Geometry: final body of the model. Coordinates: model frame, mm. Face numbers are marked on the shaded views. A direction names the side the tool comes from. Give positions to 0.01 mm unless a question says otherwise; leave off trailing zeros. Write each loop counter-clockwise with the first axis right and the second up, starting at its lowest first coordinate (ties: lowest second). Pieces come first, ordered by that corner, then holes.
Q1. Line query: line 1 (X direction, y = 0, z = 16.25); line 2 (Y direction, x = -2, z = 49); line 3 (Y direction, x = 0, z = 36). Output: solid intervals per line, ascending.
Q2. Section B-B (y = -64). Return the cut outline in (x, z).
Q3. Pin query (flat end, axial travel): pin 1 Ø22 at (x, z) = (-65, 62.5) entering from -Y; pin 2 Ø3 at (x, z) = (-22.5, 46.5) entering from +Y; pin 3 Ø13 at (x, y) = (50, 50) entering from +Z; pin 4 Ø1 at (x, y) = (-41.5, -2) entering from -Z. Return the tip coordinate at first contact, or that it passes through.
Q4. Mould query, pull axis X, two halves, no side actions, for the marked faces 1, 2, 3 and 4. Classes: +X half, -X half, draft (parallel to the pull), parting line (faces both ways), or undercut.
Q5. Section A-A (x = -91.5). Return the cut outline in (y, z), plus the area to 3 significant figures.
Q6. Section D-D (x = -46). Return the cut outline in (y, z), plus the area to 3 significant figures.
Q7. Reachability of the marked faces 5, 6 and 7 from +Z, -Z, +X, -X, +Y, -Y: full face, straight path, thin tool, end or side. Return the list, or none.
Q8. Section C-C (z = 63.5). Return the cut outline in (x, y), plus the area to 3 significant figures.
from build123d import *
from build123d.topology import SkipClean

# Parameters (mm, degrees)
SKETCH1_R           = 110
BOSS_EXTRUDE2_DEPTH = 50
SKETCH3_R           = 100
CUT_EXTRUDE1_DEPTH  = 30
SKETCH4_R           = 10
SKETCH4_R_2         = 5
CUT_EXTRUDE2_DEPTH  = 20
CUT_EXTRUDE3_DEPTH  = 10
BOSS_EXTRUDE3_START = 20
BOSS_EXTRUDE3_DEPTH = 20
CUT_EXTRUDE6_START  = -30
CUT_EXTRUDE6_DEPTH  = 30
BOSS_EXTRUDE4_DEPTH = 20
BOSS_EXTRUDE5_DEPTH = 20
BOSS_EXTRUDE6_DEPTH = 30
CUT_EXTRUDE8_START  = -30
SKETCH11_R          = 5
CUT_EXTRUDE8_DEPTH  = 30
CUT_EXTRUDE9_START  = -50
SKETCH12_R          = 5
CUT_EXTRUDE9_DEPTH  = 50
CUT_EXTRUDE10_START = -50
SKETCH13_R          = 5
CUT_EXTRUDE10_DEPTH = 50


with BuildPart() as part:
    # Sketch1 → Boss-Extrude2 (new body)
    with BuildSketch(Plane.XY):
        Circle(SKETCH1_R)
    extrude(amount=BOSS_EXTRUDE2_DEPTH)

    # Sketch3 → Cut-Extrude1 (cut)
    with BuildSketch(Plane(origin=(0, 0, 0), x_dir=(-1, 0, 0), z_dir=(0, 0, -1))):
        Circle(SKETCH3_R)
    extrude(amount=-CUT_EXTRUDE1_DEPTH, mode=Mode.SUBTRACT)

    # Sketch4 → Cut-Extrude2 (cut)
    with BuildSketch(Plane.XY.offset(50)):
        Circle(SKETCH4_R)
        with Locations((-50, 0)):
            Circle(SKETCH4_R)
        with Locations((35, 0)):
            Circle(SKETCH4_R_2)
    extrude(amount=-CUT_EXTRUDE2_DEPTH, mode=Mode.SUBTRACT)

    # Sketch5 → Cut-Extrude3 (cut)
    with BuildSketch(Plane.XY.offset(50)):
        with BuildLine():
            Line((-50, 20), (0, 20))
            ThreePointArc((0, 20), (20, 0), (0, -20))
            Line((0, -20), (-50, -20))
            ThreePointArc((-50, -20), (-70, 0), (-50, 20))
        make_face()
    extrude(amount=-CUT_EXTRUDE3_DEPTH, mode=Mode.SUBTRACT)

    # Sketch6 → Boss-Extrude3 (add)
    with BuildSketch(Plane.XY.offset(40).offset(BOSS_EXTRUDE3_START)):
        with BuildLine():
            Line((0, -10), (0, -20))
            ThreePointArc((0, -20), (20, 0), (0, 20))
            Line((0, 20), (0, 10))
            ThreePointArc((0, 10), (7.071067812, 7.071067812), (10, 0))
            ThreePointArc((10, 0), (7.071067812, -7.071067812), (0, -10))
        make_face()
    extrude(amount=-BOSS_EXTRUDE3_DEPTH)

    # Sketch7 → Cut-Extrude6 (cut)
    with BuildSketch(Plane.XY.offset(50).offset(CUT_EXTRUDE6_START)):
        with BuildLine():
            ThreePointArc((-105.909090909, 29.719765524), (-80, 0), (-105.909090909, -29.719765524))
            ThreePointArc((-105.909090909, -29.719765524), (-110, 0), (-105.909090909, 29.719765524))
        make_face()
    extrude(amount=CUT_EXTRUDE6_DEPTH, mode=Mode.SUBTRACT)

    # Sketch8 → Boss-Extrude4 (add)
    with BuildSketch(Plane.XY.offset(50)):
        with BuildLine():
            Line((0, 50), (0, 80))
            ThreePointArc((0, 80), (-44.72135955, 66.332495807), (-74.161984871, 30))
            Line((-74.161984871, 30), (-40, 30))
            ThreePointArc((-40, 30), (-22.360679775, 44.72135955), (0, 50))
        make_face()
    extrude(amount=BOSS_EXTRUDE4_DEPTH)

    # Sketch9 → Boss-Extrude5 (add)
    with BuildSketch(Plane.XY.offset(50)):
        with BuildLine():
            Line((0, -50), (0, -80))
            ThreePointArc((0, -80), (-44.72135955, -66.332495807), (-74.161984871, -30))
            Line((-74.161984871, -30), (-40, -30))
            ThreePointArc((-40, -30), (-22.360679775, -44.72135955), (0, -50))
        make_face()
    extrude(amount=BOSS_EXTRUDE5_DEPTH)

    # Sketch10 → Boss-Extrude6 (add)
    with SkipClean():  # the faces are left unmerged after this step: merging them gives an invalid solid
        with BuildSketch(Plane.XY.offset(50)):
            with BuildLine():
                Line((0, 80), (0, 50))
                ThreePointArc((0, 50), (50, 0), (0, -50))
                Line((0, -50), (0, -80))
                ThreePointArc((0, -80), (80, 0), (0, 80))
            make_face()
        extrude(amount=BOSS_EXTRUDE6_DEPTH)
    add(part.part.scale(1), mode=Mode.REPLACE)  # the faces are merged on a copy

    # Sketch11 → Cut-Extrude8 (cut)
    # profile 1 of 2: a face of its own
    with BuildSketch(Plane.XY.offset(80).offset(CUT_EXTRUDE8_START)):
        with BuildLine():
            ThreePointArc((43.816047842, -66.933952158), (55.693458652, -57.430293951), (65.557268925, -45.850239816))
            Line((65.557268925, -45.850239816), (62.096867875, -41.130626425))
            ThreePointArc((62.096867875, -41.130626425), (41.130626425, -37.903132125), (37.903132125, -58.869373575))
            Line((37.903132125, -58.869373575), (43.816047842, -66.933952158))
        make_face()
        with Locations((50, -50)):
            Circle(SKETCH11_R, mode=Mode.SUBTRACT)
    # profile 2 of 2: a face of its own
    with BuildSketch(Plane.XY.offset(80).offset(CUT_EXTRUDE8_START)):
        with BuildLine():
            Line((43.816047842, 66.933952158), (37.903132125, 58.869373575))
            ThreePointArc((37.903132125, 58.869373575), (40.679714776, 38.247030872), (61.392272116, 40.242124409))
            Line((61.392272116, 40.242124409), (65.531313117, 45.887329418))
            ThreePointArc((65.531313117, 45.887329418), (55.67720736, 57.446049304), (43.816047842, 66.933952158))
        make_face()
        with Locations((50, 50)):
            Circle(SKETCH11_R, mode=Mode.SUBTRACT)
    extrude(amount=CUT_EXTRUDE8_DEPTH, mode=Mode.SUBTRACT)

    # Sketch12 → Cut-Extrude9 (cut)
    with SkipClean():  # the faces are left unmerged after this step: merging them gives an invalid solid
        with BuildSketch(Plane.XY.offset(80).offset(CUT_EXTRUDE9_START)):
            with Locations((50, 50)):
                Circle(SKETCH12_R)
        extrude(amount=CUT_EXTRUDE9_DEPTH, mode=Mode.SUBTRACT)

    # Sketch13 → Cut-Extrude10 (cut)
    with SkipClean():  # the faces are left unmerged after this step: merging them gives an invalid solid
        with BuildSketch(Plane.XY.offset(80).offset(CUT_EXTRUDE10_START)):
            with Locations((50, -50)):
                Circle(SKETCH13_R)
        extrude(amount=CUT_EXTRUDE10_DEPTH, mode=Mode.SUBTRACT)


solid = part.part
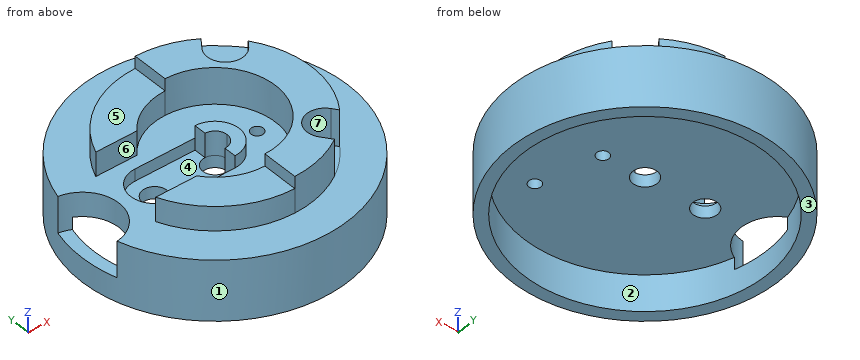
Computed:
1. line 1: x = -110 to -100, 100 to 110
1. line 2: y = -109.98 to -20, 20 to 109.98
1. line 3: y = -110 to -10, 10 to 110
2. outline: (-89.47, 0) - (-76.84, 0) - (-76.84, 30) - (76.84, 30) - (76.84, 0) - (89.47, 0) - (89.47, 50) - (41.66, 50) - (41.66, 80) - (0, 80) - (0, 70) - (-48, 70) - (-48, 50) - (-89.47, 50) - close
3. pin 1: stops at y = -59.03
3. pin 2: stops at y = 107.98
3. pin 3: stops at z = 50
3. pin 4: passes through
4. face 1: parting line
4. face 2: undercut
4. face 3: draft
4. face 4: undercut
5. outline: (-61.06, 0) - (-40.35, 0) - (-40.35, 30) - (-23.62, 30) - (-23.62, 50) - (-61.06, 50) - close; (23.62, 30) - (40.35, 30) - (40.35, 0) - (61.06, 0) - (61.06, 50) - (23.62, 50) - close
5. area: 2,740 mm2
6. outline: (-99.92, 0) - (-88.79, 0) - (-88.79, 30) - (-9.17, 30) - (-9.17, 40) - (-20, 40) - (-20, 50) - (-30, 50) - (-30, 70) - (-65.45, 70) - (-65.45, 50) - (-99.92, 50) - close; (9.17, 30) - (88.79, 30) - (88.79, 0) - (99.92, 0) - (99.92, 50) - (65.45, 50) - (65.45, 70) - (30, 70) - (30, 50) - (20, 50) - (20, 40) - (9.17, 40) - close
6. area: 5,500 mm2
7. face 5: +Z, -X, +Y, -Y
7. face 6: +Z, -X
7. face 7: +Z
8. outline: (-74.16, -30) arc R80 ccw to (43.82, -66.93) - (37.9, -58.87) arc R15 cw to (62.1, -41.13) - (65.56, -45.85) arc R80 ccw to (65.53, 45.89) - (61.39, 40.24) arc R15 cw to (37.9, 58.87) - (43.82, 66.93) arc R80 ccw to (-74.16, 30) - (-40, 30) arc R50 cw (long way) to (-40, -30) - close
8. area: 9,140 mm2
